Verification items for this drawing (mm, ordinates from the low corner). A direction names the side the tool comes from. Round coordinates to 2 decimals unless told otherwise and drop trailing zeros. Write each loop counter-clockwise with the first axis right and the second up, starting at its lowest first coordinate (ties: lowest second). Pieces come first, ordered by that corner, then holes.
Item 1: Access from +Z, -Z, +X, -X, +Y, -Y to the whole of each face (thin tool, end or side, straight path). Record for the marked faces 1, 2, 3, 4 and 5.
Item 2: Cross-section at A-A (y = 15). Enter the section's corners in (x, z), then the cut area to 3 significant figures.
Item 3: Cross-section at B-B (z = 2.1). Enter the section's corners in (x, y), then the cut area to 3 significant figures.
Item 4: Cross-section at C-C (x = 10.75). Enter the section's corners in (y, z), then the cut area to 3 significant figures.
Item 5: Scan lines: probe 1 along X at (y, z) = (1.25, 0.6); probe 2 along Y at (x, z) = (10.25, 2.4). Record each from-to range of solid material in increasing order.
Item 6: Draft check along X on the marked faces 6, 7, 8 and 9. Enter one of: pulls with the +X half, pulls with the -X half, needs draft (parallel to the pull), parting line crosses it, or undercut.
Item 7: Depth check by flat-ended pin: P1, Ø0.9, axis at y = 1.5, z = 2, coming from the +X side; P2, Ø1.6, axis at x = 1, z = 1.5, coming from the +Y side; P3, Ø0.6, axis at x = 24, z = 1.5, coming from the -Y side; P4, Ø1.5, axis at y = 9.5, z = 1, coming from the -X side. Enter the tip coordinate at first touch or a pass-through.
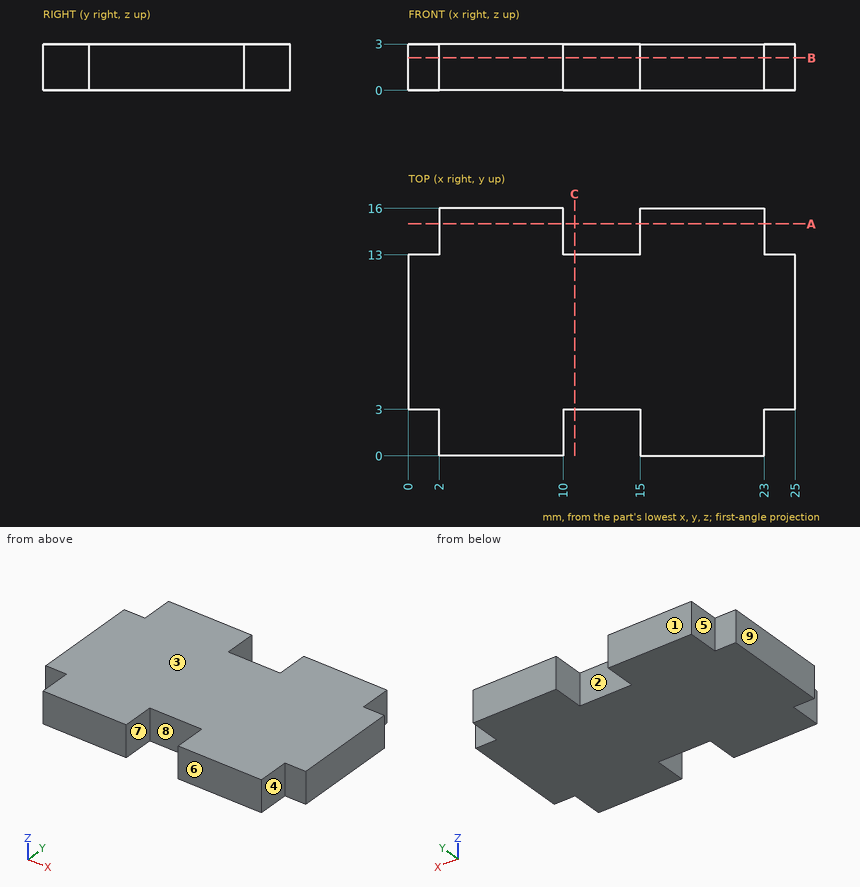
Resolved:
1. face 1: +Z, -Z, +X, -X, +Y
1. face 2: +Z, -Z, +Y
1. face 3: +Z, +X, -X, +Y, -Y
1. face 4: +Z, -Z, +X, -Y
1. face 5: +Z, -Z, -X, +Y
2. outline: (2, 0) - (10, 0) - (10, 3) - (2, 3) - close; (15, 0) - (23, 0) - (23, 3) - (15, 3) - close
2. area: 48.0 mm2
3. outline: (0, 3) - (2, 3) - (2, 0) - (10, 0) - (10, 3) - (15, 3) - (15, 0) - (23, 0) - (23, 3) - (25, 3) - (25, 13) - (23, 13) - (23, 16) - (15, 16) - (15, 13) - (10, 13) - (10, 16) - (2, 16) - (2, 13) - (0, 13) - close
3. area: 346 mm2
4. outline: (3, 0) - (13, 0) - (13, 3) - (3, 3) - close
4. area: 30.0 mm2
5. probe 1: x = 2 to 10, 15 to 23
5. probe 2: y = 3 to 13
6. face 6: needs draft
6. face 7: undercut
6. face 8: undercut
6. face 9: pulls with the -X half
7. P1: stops at x = 23
7. P2: stops at y = 13
7. P3: stops at y = 3
7. P4: stops at x = 0
